Here's how the part is built. I have some questions about the finished solid (model axes, mm). Round coordinates to 2 decimals unless told otherwise and drop trailing zeros. Write each loop counter-clockwise with the first axis right and the second up, starting at its lowest first coordinate (ties: lowest second). Pieces come first, ordered by that corner, then holes. Notation, with made-up numbers: (60, 58) - (69, 58) arc R14 cw to (69, 66) - close; hole circle Ø7 at (56, 85.5). An arc over 180 degrees is marked (long way). One line per item, written item: value. Start each with the question number.
Item 1: Imagine slicing it at C-C, the plane y = -2.95. Please give me the cut outline in (x, z).
Item 2: Imagine slicing it at B-B, the plane z = 1. Count the separate pieces of the cut face and the enclosed holes in it, then the cut area to 3 significant figures.
Item 3: If I drill on line 1 (X direction, y = -14, z = 0.35); line 2 (Y direction, x = 14.5, z = 0.25); line 3 (Y direction, x = -13.5, z = 0.5), over which ranges is the centre line in solid material (lowest first)?
Item 4: For P1, Ø1, axis at x = -20.5, z = 0.5, coming from the -Y side; P2, Ø1, axis at y = -29.5, z = 0.5, coming from the +X side, each with a flat end and sliding along its axis, tell me the tip position at first contact or that it passes through.
Item 5: Imagine slicing it at A-A, the plane y = -19.5. Please give me the cut outline in (x, z), then the cut area to 3 significant figures.
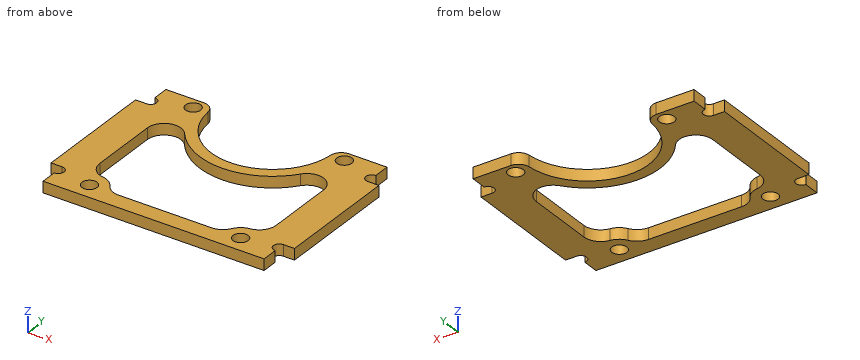
Autodesk Inventor part; units mm, degrees
ref_plane "YZ Plane" through (0, 0, 0) normal (1, 0, 0) x (0, 1, 0)
ref_plane "XZ Plane" through (0, 0, 0) normal (0, 1, 0) x (-1, 0, 0)
ref_plane "XY Plane" through (0, 0, 0) normal (0, 0, 1) x (1, 0, 0)
sketch "スケッチ1" plane through (0, 0, 0) normal (0, 0, 1) x (1, 0, 0)
  circle A0 centre (0, 0) radius 10.5 construction
  line L0 (-13.5, -1) -> (13.5, -1) construction
  line L1 (13.5, -1) -> (13.5, -28) construction
  line L2 (13.5, -28) -> (-13.5, -28) construction
  line L3 (-13.5, -28) -> (-13.5, -1) construction
  circle A1 centre (-13.5, -1) radius 1.35
  circle A2 centre (13.5, -1) radius 1.35
  circle A3 centre (-13.5, -28) radius 1.35
  circle A4 centre (13.5, -28) radius 1.35
  line L4 (-19.75, 1) -> (-19.75, -1.9)
  line L5 (-19.75, -4) -> (-21.75, -4)
  line L6 (-21.75, -4) -> (-21.75, -26)
  line L7 (-21.75, -26) -> (-19.75, -26)
  line L8 (-19.75, -28.1) -> (-19.75, -31)
  line L9 (-19.75, -31) -> (19.75, -31)
  line L10 (19.75, -31) -> (19.75, -28.1)
  line L11 (19.75, -4) -> (21.75, -4)
  line L12 (21.75, -4) -> (21.75, -26)
  line L13 (21.75, -26) -> (19.75, -26)
  line L14 (0, 0) -> (0, -28) construction
  line L15 (-21.75, -15) -> (21.75, -15) construction
  arc A5 (-19.75, -4) -> (-19.75, -1.9) centre (-19.75, -2.95) ccw
  line L16 (-19.75, 1) -> (-10.9545, 1)
  circle A6 centre (-13.5, -1) radius 2 construction
  arc A7 (-19.75, -28.1) -> (-19.75, -26) centre (-19.75, -27.05) ccw
  arc A8 (19.75, -26) -> (19.75, -28.1) centre (19.75, -27.05) ccw
  line L17 (10.9545, 1) -> (19.75, 1)
  line L18 (19.75, 1) -> (19.75, -1.9)
  arc A9 (19.75, -1.9) -> (19.75, -4) centre (19.75, -2.95) ccw
  arc A10 (-10.9545, 1) -> (10.9545, 1) centre (0, 0) ccw
  point P0 (0, -1)
  dimension "d0" = 21
  dimension "d1" = 1
  dimension "d2" = 27
  dimension "d3" = 2.7
  dimension "d6" = 27
  dimension "d9" = 27
  dimension "d12" = 15
  dimension "d27" = 22
  dimension "d35" = 2
  dimension "d37" = 1.05
  dimension "d41" = 5
  dimension "d42" = 4
  dimension "d43" = 0.5
  dimension "d44" = 39.5
extrude "押し出し1" add sketch "スケッチ1" along normal blind 2
sketch "スケッチ2" plane through (0, 0, 2) normal (0, 0, 1) x (1, 0, 0)
  circle A0 centre (13.5, -28) radius 1.35
  circle A1 centre (-13.5, -28) radius 1.35
  circle A2 centre (13.5, -1) radius 1.35
  circle A3 centre (-13.5, -1) radius 1.35
  line L0 (-19.75, 1) -> (-19.75, -1.9)
  line L1 (-19.75, -31) -> (19.75, -31)
  arc A4 (-10.9545, 1) -> (10.9545, 1) centre (0, 0) ccw
  line L2 (-15.75, -2.9843) -> (-15.75, -25)
  line L3 (-15.75, -25) -> (-13.5, -25)
  arc A5 (-10.5, -28) -> (-13.5, -25) centre (-13.5, -28) ccw
  arc A6 (-15.75, -2.9843) -> (-12.4312, -3.8032) centre (-13.5, -1) ccw
  arc A7 (-12.4312, -3.8032) -> (12.4312, -3.8032) centre (0, 0) ccw
  arc A8 (12.4312, -3.8032) -> (15.75, -2.9843) centre (13.5, -1) ccw
  line L4 (15.75, -2.9843) -> (15.75, -25)
  line L5 (15.75, -25) -> (13.5, -25)
  arc A9 (13.5, -25) -> (10.5, -28) centre (13.5, -28) ccw
  line L6 (-10.5, -28) -> (10.5, -28)
  line L7 (0, 0) -> (0, -31) construction
  dimension "d47" = 3
  dimension "d48" = 4
  dimension "d49" = 2
  dimension "d50" = 3
extrude "押し出し2" cut sketch "スケッチ2" against normal blind 10 contours A6 A7 A8 L4 L5 A9 L6 A5 L3 L2
fillet "フィレット1" radius 3 8 edges at (-15.75, -2.9843, 1) (-12.4312, -3.8032, 1) (15.75, -2.9843, 1) (12.4312, -3.8032, 1) (-15.75, -25, 1) (-10.5, -28, 1) (15.75, -25, 1) (10.5, -28, 1)
fillet "フィレット1" radius 2 2 edges at (-10.9545, 1, 1) (10.9545, 1, 1)
equation "\"d6\" = d2"
equation "\"d9\" = d2"
equation "\"d27\" = d17"
equation "\"d41\" = d18"
properties part number "付け根_サブフレーム_1_1" material "アルミニウム 2014-T4"
Values follow:
1. outline: (-18.7, 0) - (-10.6, 0) - (-10.6, 2) - (-18.7, 2) - close; (10.6, 0) - (18.7, 0) - (18.7, 2) - (10.6, 2) - close
2. separate pieces: 1
2. enclosed holes: 5
2. area: 574 mm^2
3. line 1: x = -21.75 to -15.75, 15.75 to 21.75
3. line 2: y = -31 to -28.91, -27.09 to -24.48, -7.23 to -1.91, -0.09 to 1
3. line 3: y = -31 to -29.35, -26.65 to -24.95, -6.76 to -2.35, 0.35 to 1
4. P1: stops at y = -26
4. P2: stops at x = 19.75
5. outline: (-21.75, 0) - (-15.75, 0) - (-15.75, 2) - (-21.75, 2) - close; (15.75, 0) - (21.75, 0) - (21.75, 2) - (15.75, 2) - close
5. area: 24.0 mm^2
